Model file for the job. Use its own axes, mm. Face numbers are marked on the shaded views. A direction names the side the tool comes from. Give positions to 0.01 mm unless a question says otherwise; leave off trailing zeros. Loops run counter-clockwise (first coordinate to the right, second up) from the corner with the lowest first, then second, coordinate; pieces in that order, holes last. Notation, with made-up numbers: M 16.5,22 L 39.5,22 A22 ccw 39.5,42 Z; hole C -31.5,83 d11. An arc over 180 degrees is marked long. Answer in a Markdown table with one row per item.
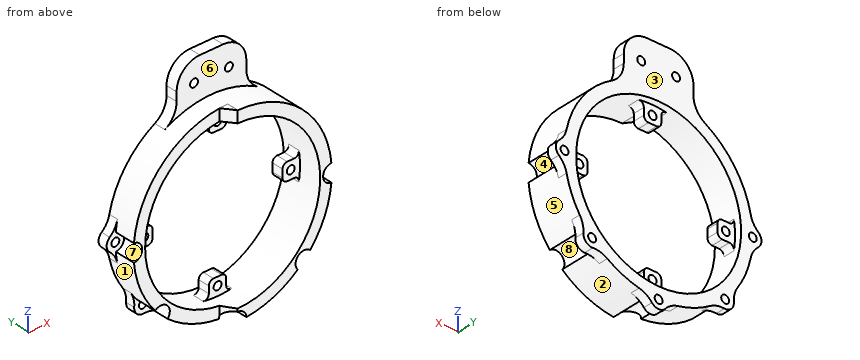
```python
from build123d import *

# Parameters (mm, degrees)
CROQUIS1_R                                           = 40.5
CROQUIS1_R_2                                         = 35.5
SALIENTE_EXTRUIR1_DEPTH                              = 9
CROQUIS2_R                                           = 1.7
SALIENTE_EXTRUIR2_DEPTH                              = 5
REDONDEO1_R                                          = 10
CROQUIS4_R                                           = 1.7
SALIENTE_EXTRUIR3_DEPTH                              = 5
REDONDEO2_R                                          = 2
MATRIZC1_COUNT                                       = 4
REDONDEO2_OF_MATRIZC1_R                              = 2
REFRENTADO_PARA_TORNILLO_CON_CABEZA_PLAN_D           = 3.4
REFRENTADO_PARA_TORNILLO_CON_CABEZA_PLAN_CBORE_D     = 7.5
REFRENTADO_PARA_TORNILLO_CON_CABEZA_PLAN_CBORE_DEPTH = 14
CROQUIS8_R                                           = 3.75
CROQUIS8_R_2                                         = 1.7
SALIENTE_EXTRUIR4_DEPTH                              = 4
MATRIZC2_COUNT                                       = 3
MATRIZC2_ANGLE                                       = 90
SIMETR_A1_COPY_1_D                                   = 3.4
SIMETR_A1_COPY_1_CBORE_D                             = 7.5
SIMETR_A1_COPY_1_CBORE_DEPTH                         = 14
SIMETR_A1_COPY_2_D                                   = 3.4
SIMETR_A1_COPY_2_CBORE_D                             = 7.5
SIMETR_A1_COPY_2_CBORE_DEPTH                         = 14
SIMETR_A1_COPY_3_SKETCH_R                            = 3.75
SIMETR_A1_COPY_3_SKETCH_R_2                          = 1.7
SIMETR_A1_COPY_3_DEPTH                               = 4
SIMETR_A1_COPY_4_SKETCH_R                            = 3.75
SIMETR_A1_COPY_4_SKETCH_R_2                          = 1.7
SIMETR_A1_COPY_4_DEPTH                               = 4
SIMETR_A1_COPY_5_D                                   = 3.4
SIMETR_A1_COPY_5_CBORE_D                             = 7.5
SIMETR_A1_COPY_5_CBORE_DEPTH                         = 14
SIMETR_A1_COPY_6_SKETCH_R                            = 3.75
SIMETR_A1_COPY_6_SKETCH_R_2                          = 1.7
SIMETR_A1_COPY_6_DEPTH                               = 4
REDONDEO3_R                                          = 10
CORTAR_EXTRUIR2_START                                = -5
CORTAR_EXTRUIR2_DEPTH                                = 5
CHAFL_N2_SIZE2                                       = 5
CHAFL_N2_SIZE                                        = 3.501037691


# Some blends are built 0.0001 mm under size
with BuildPart() as part:
    # Croquis1 → Saliente-Extruir1 (new, symmetric)
    with BuildSketch(Plane(origin=(0, 0, 0), x_dir=(1, 0, 0), z_dir=(0, 1, 0))):
        with Locations(Location((0, 0, 0), (0, 0, 270))):
            Circle(CROQUIS1_R)
        with Locations(Location((0, 0, 0), (0, 0, 270))):
            Circle(CROQUIS1_R_2, mode=Mode.SUBTRACT)
    extrude(amount=SALIENTE_EXTRUIR1_DEPTH, both=True)

    # Croquis2 → Saliente-Extruir2 (add)
    with BuildSketch(Plane.XZ.offset(-9)):
        with BuildLine():
            Line((-15, 37.619808612), (-15, 57.619808612))
            Line((-15, 57.619808612), (15, 57.619808612))
            Line((15, 57.619808612), (15, 37.619808612))
            ThreePointArc((15, 37.619808612), (0, 40.5), (-15, 37.619808612))
        make_face()
        with Locations(Location((-7.5, 47.916594203, 0), (0, 0, 270))):
            Circle(CROQUIS2_R, mode=Mode.SUBTRACT)
        with Locations(Location((7.5, 47.916594203, 0), (0, 0, 90))):
            Circle(CROQUIS2_R, mode=Mode.SUBTRACT)
    extrude(amount=SALIENTE_EXTRUIR2_DEPTH)

    # Redondeo1
    redondeo1_edges = [part.edges().sort_by_distance(p)[0] for p in [
        (-15, 6.5, 37.619808612),
        (15, 6.5, 37.619808612),
        (15, 6.5, 57.619808612),
        (-15, 6.5, 57.619808612),
    ]]
    fillet(redondeo1_edges, radius=REDONDEO1_R)

    # Croquis4 → Saliente-Extruir3 (add)
    with BuildSketch(Plane(origin=(0, 1, 0), x_dir=(-1, 0, 0), z_dir=(0, -1, 0))):
        with BuildLine():
            Line((-3.75, -35.301380993), (-3.75, -28))
            Line((-3.75, -28), (3.75, -28))
            Line((3.75, -28), (3.75, -35.301380993))
            ThreePointArc((3.75, -35.301380993), (0, -35.5), (-3.75, -35.301380993))
        make_face()
        with Locations(Location((0, -31.5, 0), (0, 0, 90))):
            Circle(CROQUIS4_R, mode=Mode.SUBTRACT)
    saliente_extruir3 = extrude(amount=-SALIENTE_EXTRUIR3_DEPTH)

    # Redondeo2
    redondeo2_edges = [part.edges().sort_by_distance(p)[0] for p in [
        (-3.75, 3.5, 35.301380993),
        (3.75, 3.5, 35.301380993),
        (3.75, 3.5, 28),
        (-3.75, 3.5, 28),
    ]]
    fillet(redondeo2_edges, radius=REDONDEO2_R)

    # MatrizC1: Saliente-Extruir3 ×4 about axis
    matrizc1_axis = Axis((0, 0, 0), (0, 1, 0))
    for i in range(1, MATRIZC1_COUNT):
        add(saliente_extruir3.rotate(matrizc1_axis, i * 360 / MATRIZC1_COUNT))

    # Redondeo2 of MatrizC1
    redondeo2_of_matrizc1_edges = [part.edges().sort_by_distance(p)[0] for p in [
        (35.301380993, 3.5, 3.75),
        (35.301380993, 3.5, -3.75),
        (28, 3.5, -3.75),
        (28, 3.5, 3.75),
        (3.75, 3.5, -35.301380993),
        (-3.75, 3.5, -35.301380993),
        (-3.75, 3.5, -28),
        (3.75, 3.5, -28),
        (-35.301380993, 3.5, -3.75),
        (-35.301380993, 3.5, 3.75),
        (-28, 3.5, 3.75),
        (-28, 3.5, -3.75),
    ]]
    fillet(redondeo2_of_matrizc1_edges, radius=REDONDEO2_OF_MATRIZC1_R)

    # Refrentado para tornillo con cabeza plana de M31 (through all)
    with Locations(Plane(origin=(0, -9, 0), x_dir=(-1, 0, 0), z_dir=(0, -1, 0))):
        with Locations((0, 40.5)):
            refrentado_para_tornillo_con_cabeza_plan = CounterBoreHole(REFRENTADO_PARA_TORNILLO_CON_CABEZA_PLAN_D / 2, REFRENTADO_PARA_TORNILLO_CON_CABEZA_PLAN_CBORE_D / 2, REFRENTADO_PARA_TORNILLO_CON_CABEZA_PLAN_CBORE_DEPTH)

    # Croquis8 → Saliente-Extruir4 (add)
    with BuildSketch(Plane(origin=(0, 9, 0), x_dir=(1, 0, 0), z_dir=(0, 1, 0))):
        with Locations((0, 40.5)):
            Circle(CROQUIS8_R)
        with Locations(Location((0, 40.5, 0), (0, 0, 90))):
            Circle(CROQUIS8_R_2, mode=Mode.SUBTRACT)
    saliente_extruir4 = extrude(amount=-SALIENTE_EXTRUIR4_DEPTH)

    # MatrizC2: Refrentado para tornillo con cabeza plana de M31, Saliente-Extruir4 ×3 about axis
    matrizc2_axis = Axis((0, 0, 0), (0, 1, 0))
    add([refrentado_para_tornillo_con_cabeza_plan.rotate(matrizc2_axis, i * MATRIZC2_ANGLE / (MATRIZC2_COUNT - 1)) for i in range(1, MATRIZC2_COUNT)], mode=Mode.SUBTRACT)
    add([saliente_extruir4.rotate(matrizc2_axis, i * MATRIZC2_ANGLE / (MATRIZC2_COUNT - 1)) for i in range(1, MATRIZC2_COUNT)])

    # Simetría1 copy 1 (through all)
    with Locations(Plane(origin=(0, -9, 0), x_dir=(0.7071067811865462, 0, 0.7071067811865488), z_dir=(0, -1, 0))):
        with Locations((0, -40.5)):
            CounterBoreHole(SIMETR_A1_COPY_1_D / 2, SIMETR_A1_COPY_1_CBORE_D / 2, SIMETR_A1_COPY_1_CBORE_DEPTH)

    # Simetría1 copy 2 (through all)
    with Locations(Plane(origin=(0, -9, 0), x_dir=(0, 0, 1), z_dir=(0, -1, 0))):
        with Locations((0, -40.5)):
            CounterBoreHole(SIMETR_A1_COPY_2_D / 2, SIMETR_A1_COPY_2_CBORE_D / 2, SIMETR_A1_COPY_2_CBORE_DEPTH)

    # Simetría1 copy 3 sketch → Simetría1 copy 3 (add)
    with BuildSketch(Plane(origin=(0, 9, 0), x_dir=(-0.7071067811865462, 0, -0.7071067811865488), z_dir=(0, 1, 0))):
        with Locations((0, -40.5)):
            Circle(SIMETR_A1_COPY_3_SKETCH_R)
        with Locations((0, -40.5)):
            Circle(SIMETR_A1_COPY_3_SKETCH_R_2, mode=Mode.SUBTRACT)
    extrude(amount=-SIMETR_A1_COPY_3_DEPTH)

    # Simetría1 copy 4 sketch → Simetría1 copy 4 (add)
    with BuildSketch(Plane(origin=(0, 9, 0), x_dir=(0, 0, -1), z_dir=(0, 1, 0))):
        with Locations((0, -40.5)):
            Circle(SIMETR_A1_COPY_4_SKETCH_R)
        with Locations((0, -40.5)):
            Circle(SIMETR_A1_COPY_4_SKETCH_R_2, mode=Mode.SUBTRACT)
    extrude(amount=-SIMETR_A1_COPY_4_DEPTH)

    # Simetría1 copy 5 (through all)
    with Locations(Plane.XZ.offset(9)):
        with Locations((0, -40.5)):
            CounterBoreHole(SIMETR_A1_COPY_5_D / 2, SIMETR_A1_COPY_5_CBORE_D / 2, SIMETR_A1_COPY_5_CBORE_DEPTH)

    # Simetría1 copy 6 sketch → Simetría1 copy 6 (add)
    with BuildSketch(Plane(origin=(0, 9, 0), x_dir=(-1, 0, 0), z_dir=(0, 1, 0))):
        with Locations((0, -40.5)):
            Circle(SIMETR_A1_COPY_6_SKETCH_R)
        with Locations((0, -40.5)):
            Circle(SIMETR_A1_COPY_6_SKETCH_R_2, mode=Mode.SUBTRACT)
    extrude(amount=-SIMETR_A1_COPY_6_DEPTH)

    # Redondeo3
    # the kernel refuses this fillet: 10 mm, written as the material it adds along each edge
    with BuildSketch(Plane(origin=(3.745979069, 5, -40.326388889), x_dir=(-0.3229702045586981, 0, -0.9464091329690941), z_dir=(0, 1, 0)), Plane(origin=(-25.866255843, 5, -31.163870246), x_dir=(-0.8975867374639902, 0, -0.4408378939346639), z_dir=(0, 1, 0)), Plane(origin=(-40.326388889, 5, -3.745979069), x_dir=(-0.9464091329690931, 0, 0.3229702045587014), z_dir=(0, 1, 0)), Plane(origin=(31.163870246, 5, -25.866255843), x_dir=(0.4408378939346665, 0, -0.897586737463989), z_dir=(0, 1, 0)), Plane(origin=(40.326388889, 5, 3.745979069), x_dir=(0.9464091329690957, 0, -0.32297020455869396), z_dir=(0, 1, 0))) as redondeo3_piece_1:
        with BuildLine():
            CenterArc((6.412684914, -9.30442023), REDONDEO3_R, 111.496176577, 37.683075119)
            ThreePointArc((-2.175059251, -4.180881398), (-1.026664082, -2.122105354), (0, 0))
            ThreePointArc((0, 0), (1.374146767, -0.260842414), (2.748293534, 0))
        make_face()
    extrude(amount=4)
    with BuildSketch(Plane(origin=(-3.745979069, 5, -40.326388889), x_dir=(-0.9886449734760148, 0, 0.15027014480797551), z_dir=(0, 1, 0)), Plane(origin=(-31.163870246, 5, -25.866255843), x_dir=(-0.5928205265272785, 0, 0.80533460333449), z_dir=(0, 1, 0)), Plane(origin=(25.866255843, 5, -31.163870246), x_dir=(-0.8053346033344878, 0, -0.5928205265272815), z_dir=(0, 1, 0)), Plane(origin=(40.326388889, 5, -3.745979069), x_dir=(-0.15027014480797213, 0, -0.9886449734760153), z_dir=(0, 1, 0))) as redondeo3_piece_2:
        with BuildLine():
            CenterArc((5.294647205, -9.98305938), REDONDEO3_R, 93.33552043, 37.683075119)
            ThreePointArc((-1.268392176, -2.438093238), (-0.402794996, -1.339430586), (0, 0))
            ThreePointArc((0, 0), (2.356408921, -0.068609509), (4.712817842, 0))
        make_face()
    extrude(amount=4)
    with BuildSketch(Plane(origin=(-40.326388889, 5, 3.745979069), x_dir=(-0.9464091329690953, 0, -0.322970204558695), z_dir=(0, 1, 0))) as redondeo3_piece_3:
        with BuildLine():
            CenterArc((6.412684914, 9.30442023), REDONDEO3_R, 210.820748304, 37.683075119)
            ThreePointArc((-2.175059251, 4.180881398), (-1.026664082, 2.122105354), (0, 0))
            ThreePointArc((0, 0), (1.374146767, 0.260842414), (2.748293534, 0))
        make_face()
    extrude(amount=4)

    # Croquis10 → Cortar-Extruir2 (cut)
    with BuildSketch(Plane.XZ.offset(9).offset(CORTAR_EXTRUIR2_START)):
        with BuildLine():
            Line((0, 40.5), (0, 35.5))
            ThreePointArc((0, 35.5), (-35.5, 0), (0, -35.5))
            Line((0, -35.5), (0, -40.5))
            ThreePointArc((0, -40.5), (-40.5, 0), (0, 40.5))
        make_face()
    extrude(amount=CORTAR_EXTRUIR2_DEPTH, mode=Mode.SUBTRACT)

    # Chaflán2
    chafl_n2_edges = [part.edges().sort_by_distance(p)[0] for p in [
        (0, -4, -36.125),
    ]]
    chafl_n2_side = [part.faces().sort_by_distance(p)[0] for p in [
        (-0.070020754, -4, -36.125),
    ]]
    chamfer(chafl_n2_edges, length=CHAFL_N2_SIZE - 0.0001, length2=CHAFL_N2_SIZE2 - 0.0001, reference=chafl_n2_side[0])  # a hair under: the kernel refuses the full size
    # the kernel refuses this chamfer: 5, 3.501037691 mm, written as the material it adds along each edge
    with BuildSketch(Plane(origin=(0, -4, 53.412761151), x_dir=(-0.9989750717851554, 0.04526373771402081, 0), z_dir=(0, 0, -1))) as chafl_n2_2_piece_1_section:
        with BuildLine():
            Line((3.619462668, 0), (-0.348331978, -5.153345411))
            Line((-0.348331978, -5.153345411), (-0.448229485, -5.148819037))
            ThreePointArc((-0.448229485, -5.148819037), (-0.21676464, -2.574742553), (-0.099897507, 0.004526374))
            Line((-0.099897507, 0.004526374), (0.004526374, 0.099897507))
            ThreePointArc((0.004526374, 0.099897507), (1.810549919, 0.01806626), (3.623989042, 0.099897507))
            Line((3.623989042, 0.099897507), (3.619462668, 0))
        make_face()
    chafl_n2_2_piece_1 = extrude(amount=30.825522303, mode=Mode.PRIVATE)
    chafl_n2_2_piece_1 = chafl_n2_2_piece_1 - Plane(origin=(0, -5.656570303, 0), x_dir=(0, 0, 1), z_dir=(0, -1, 0)) * Cylinder(35.5, 83, mode=Mode.PRIVATE)
    chafl_n2_2_piece_1 = chafl_n2_2_piece_1 & Plane(origin=(0, -5.656570303, 0), x_dir=(0, 0, 1), z_dir=(0, 1, 0)) * Cylinder(40.5, 83, mode=Mode.PRIVATE)
    chafl_n2_2_piece_1 = split(chafl_n2_2_piece_1, bisect_by=Plane(origin=(-1.140213067, -9, 37.972268043), z_dir=(0, 1, 0)), keep=Keep.TOP, mode=Mode.PRIVATE)
    add(chafl_n2_2_piece_1)


solid = part.part
```
(1) Flat gauge pins, fed straight in: P1, Ø2, axis at x = 32, z = 1.5, coming from the -Y side; P2, Ø18.5, axis at x = -19.5, z = -19.5, coming from the -Y side; P3, Ø0.9, axis at y = 4.5, z = 31.5, coming from the +X side. Where does each tip first touch, or does it go through?
Established:
| item | result |
|---|---|
| P1 | stops at y = 1 |
| P2 | stops at y = -4 |
| P3 | stops at x = 26 |
(2) Which spindle directions (+Z, -Z, +X, -X, +Y, -Y) get a long thin tool onto all of the face, cutting with end or side? Do the marked faces 1, 2, 3 and 4. Say none if no direction does.
Established:
| item | result |
|---|---|
| face 1 | -Z, -X, -Y |
| face 2 | -Z, +X, -Y |
| face 3 | +Z, -Z, +X, -X, +Y |
| face 4 | +X, -Y |
(3) Saw through at B-B, the plane z = 25. Give the cut face in (x, y), and give its area (3 significant figures).
Established:
| item | result |
|---|---|
| outline | M -31.86,-4 L -25.2,-4 L -25.2,9 L -31.86,9 Z; M 25.2,-9 L 31.86,-9 L 31.86,9 L 25.2,9 Z |
| area | 206 mm2 |
(4) Wall check: L1, parallel to Z at x = -31.5, y = 3.35; L2, parallel to Z at x = 7.5, y = 5; L3, parallel to X at y = -2.75, z = 17. Give the ranges that are in metal, low to high.
Established:
| item | result |
|---|---|
| L1 | z = -25.46 to -16.37, -3.75 to -1.7, 1.7 to 3.75, 16.37 to 25.46 |
| L2 | z = -39.8 to -34.7, 34.7 to 46.22, 49.62 to 57.3 |
| L3 | x = -36.76 to -31.16, 31.16 to 36.76 |
(5) Mould opens along Z. For the marked faces 5, 6, 7 and 8 say: pulls with the +Z half, pulls with the -Z half, needs draft (parallel to the pull), parting line crosses it, or undercut.
Established:
| item | result |
|---|---|
| face 5 | pulls with the -Z half |
| face 6 | needs draft |
| face 7 | undercut |
| face 8 | undercut |
(6) Saw through at C-C, the plane x = -13. Give the cut face in (y, z), and give its area (3 significant figures).
Established:
| item | result |
|---|---|
| outline | M -4,-38.36 L 9,-38.36 L 9,-33.03 L -4,-33.03 Z; M -4,33.03 L 9,33.03 L 9,53.62 L 4,53.62 L 4,38.36 L -4,38.36 Z |
| area | 215 mm2 |
(7) Saw through at A-A, the plane y = -0.5. Give the cut face in (x, z), and give its area (3 significant figures).
Established:
| item | result |
|---|---|
| outline | M -40.33,-3.75 A40.5 ccw -31.16,-25.87 A3.75 cw -25.87,-31.16 A40.5 ccw -3.75,-40.33 A3.75 cw 3.75,-40.33 A40.5 ccw 25.87,-31.16 A3.75 cw 31.16,-25.87 A40.5 ccw 40.33,-3.75 A3.75 cw 40.33,3.75 A40.5 ccw -40.33,3.75 A3.75 cw Z; hole C 0,0 d71 |
| area | 1,090 mm2 |
